Source: CAD feature listing. Evaluate the final solid. Frame: model axes, mm. A direction names the side the tool comes from. Coordinates: 2 decimals unless noted, no trailing zeros. Loops run counter-clockwise (first coordinate to the right, second up) from the corner with the lowest first, then second, coordinate; pieces in that order, holes last. Notation, with made-up numbers: M -34.75,18 L 21.25,18 A24 cw 21.25,36 Z; hole C 53.5,1.5 d10. An arc over 180 degrees is marked long. One line per question, with ' | ' between items. Start each with the question number.
1. Pin query (flat end, axial travel): P1, Ø12, axis at x = -6.5, z = -4, coming from the -Y side; P2, Ø1.4, axis at x = -0.5, y = -0.5, coming from the -Z side; P3, Ø1.5, axis at x = 5, z = 8, coming from the +Y side. Return the tip coordinate at first contact, or that it passes through.
2. Mould query, pull axis Z, two halves, no side actions, for faces 1 (the cylindrical face through (0, 2, 5)), 2 (the flat face through (3, 2, 1)), 3 (the flat face through (-2, 19, -10)), 4 (the flat face through (7, 11, -4)). Classes: pulls with the +Z half, pulls with the -Z half, needs draft (parallel to the pull), parting line crosses it, or undercut.
3. Section query B-B, the plane y = 15.5. Output: boundary loops of the cut face in (x, z).
4. Access query for faces 5 (the flat face through (0, -1, 10.1)), 6 (the flat face through (9, 26, -8)), 7 (the flat face through (3, -1, -11)), 8 (the flat face through (0, 24.1, -15)), 9 (the flat face through (-3.2, 4, 1.8)). Directions: +Z, -Z, +X, -X, +Y, -Y. A direction counts if a zero-diameter tool reaches every point of the face in a straight line with its end or side. Return the directions, or none.
5. Section query A-A, the plane x = 0. State how many separate pieces and enclosed holes the cut face has, and give its area (3 significant figures).
6. Section query C-C, the plane z = 11.25. Output: boundary loops of the cut face in (x, y), and give its area (3 significant figures).
7. Section query D-D, the plane x = 7.5. Output: boundary loops of the cut face in (y, z).
8. Ray query, probe 1 along X at (y, z) = (6.5, 6); probe 2 along X at (y, z) = (3.75, 1.25); probe 3 along Y at (x, z) = (-8.75, 6). Return the intervals inside material, ascending.
```python
from build123d import *

# Parameters (mm, degrees)
SKETCH1_W           = 20
SKETCH1_H           = 28
BOSS_EXTRUDE1_DEPTH = 4
CUT_EXTRUDE1_DEPTH  = 18.663521733
SKETCH4_W           = 6
SKETCH4_H           = 2
BOSS_EXTRUDE2_DEPTH = 1.25
MIRROR1_START       = -14
MIRROR1_OUTLINE_W   = 20
MIRROR1_OUTLINE_H   = 24
MIRROR1_DEPTH       = 4
MIRROR1_START_2     = -15.25
MIRROR1_2_OUTLINE_W = 6
MIRROR1_2_OUTLINE_H = 2
MIRROR1_2_DEPTH     = 1.25
BOSS_EXTRUDE3_DEPTH = 3


# Read off the part's stored shape, not the designer's step: Mirror1
with BuildPart() as part:
    # Sketch1 → Boss-Extrude1 (new body)
    with BuildSketch(Plane(origin=(0, 0, 0), x_dir=(1, 0, 0), z_dir=(0, 1, 0))):
        Rectangle(SKETCH1_W, SKETCH1_H)
    extrude(amount=BOSS_EXTRUDE1_DEPTH)

    # Sketch3 → Cut-Extrude1 (cut, through all)
    with BuildSketch(Plane(origin=(0, 4, 0), x_dir=(1, 0, 0), z_dir=(0, 1, 0))):
        with BuildLine():
            Line((3, 0), (3, -2))
            ThreePointArc((3, -2), (0, -5), (-3, -2))
            Line((-3, -2), (-3, 0))
            ThreePointArc((-3, 0), (0, 3), (3, 0))
        make_face()
    extrude(amount=-CUT_EXTRUDE1_DEPTH, mode=Mode.SUBTRACT)

    # Sketch4 → Boss-Extrude2 (add)
    with BuildSketch(Plane.XZ):
        with Locations((0, 11.1)):
            Rectangle(SKETCH4_W, SKETCH4_H)
        with Locations((0, -11)):
            Rectangle(SKETCH4_W, SKETCH4_H)
    extrude(amount=BOSS_EXTRUDE2_DEPTH)

    # Mirror1 outline → Mirror1 (add)
    with BuildSketch(Plane.XY.offset(MIRROR1_START)):
        with Locations((0, 16)):
            Rectangle(MIRROR1_OUTLINE_W, MIRROR1_OUTLINE_H)
        with BuildLine():
            ThreePointArc((-3, 16), (0, 19), (3, 16))
            Line((3, 16), (3, 14))
            ThreePointArc((3, 14), (0, 11), (-3, 14))
            Line((-3, 14), (-3, 16))
        make_face(mode=Mode.SUBTRACT)
    extrude(amount=MIRROR1_DEPTH)

    # Mirror1 2 outline → Mirror1 2 (add)
    with BuildSketch(Plane.XY.offset(MIRROR1_START_2)):
        with Locations((0, 3)):
            Rectangle(MIRROR1_2_OUTLINE_W, MIRROR1_2_OUTLINE_H)
        with Locations((0, 25.1)):
            Rectangle(MIRROR1_2_OUTLINE_W, MIRROR1_2_OUTLINE_H)
    extrude(amount=MIRROR1_2_DEPTH)

    # Sketch5 → Boss-Extrude3 (add)
    with BuildSketch(Plane(origin=(10, 0, 0), x_dir=(0, 0, -1), z_dir=(1, 0, 0))):
        Polygon((-14, 4), (-14, 6), (-9.5, 6), (8, 23.5), (8, 28), (10, 28), (10, 4), align=None)
    boss_extrude3 = extrude(amount=-BOSS_EXTRUDE3_DEPTH)

    # Mirror2: Boss-Extrude3 across plane
    add(boss_extrude3.mirror(Plane(origin=(0, 0, 0), x_dir=(0, 0, 1), z_dir=(1, 0, 0))))


solid = part.part
```
Taken from the geometry:
1) P1: y = 0 | P2: z = -14 | P3: y = 4
2) face 1: undercut | face 2: undercut | face 3: pulls with the +Z half | face 4: needs draft
3) outline: M -10,-14 L -3,-14 L -3,-10 L -7,-10 L -7,0 L -10,0 Z; M 3,-14 L 10,-14 L 10,0 L 7,0 L 7,-10 L 3,-10 Z
4) face 5: +X, -X, -Y | face 6: +Z, +X, -X, +Y | face 7: +Z, -Z, +X, -Y | face 8: -Z, +X, -X | face 9: +Z, +Y
5) separate pieces: 3 | enclosed holes: 0 | area: 154 mm^2
6) outline: M -10,0 L -3,0 L -3,-1.25 L 3,-1.25 L 3,0 L 10,0 L 10,6 L 7,6 L 7,4 L -7,4 L -7,6 L -10,6 Z | area: 99.5 mm^2
7) outline: M 0,-14 L 28,-14 L 28,-8 L 23.5,-8 L 6,9.5 L 6,14 L 0,14 Z
8) probe 1: -10 to -7, 7 to 10 | probe 2: -10 to -3, 3 to 10 | probe 3: 0 to 9.5
